Input: part model. Units: mm. Frame: model coordinates. A direction names the side the tool comes from. Coordinates: 2 decimals unless noted, no trailing zeros. Order: outer loops, then holes, each group sorted by start corner. A loop starts at its lowest first (then second) coordinate and runs counter-clockwise, first axis right, second up. Notation, with made-up numbers: (-24, 27) - (0, 27) arc R24 ccw to (0, 41) - close; hole circle Ø7 at (49.25, 66). An arc over 180 degrees is marked (long way). Use a Markdown table: item, result. Add a question column.
from build123d import *

# Parameters (mm, degrees)
F2_R     = 17.5
F3_DEPTH = 25
F5_SCALE = 0.5


with BuildPart() as f1:
    # F0 (on Front) → F1 (revolve)
    with BuildSketch(Plane.XZ):
        Polygon((0, 37.8452404466), (0, 0), (12.7, 0), (12.7, 52.3875), (4.4460149232, 52.3875), align=None)
        Polygon((0, 52.3875), (0, 37.8452404466), (4.4460149232, 52.3875), align=None)
        Polygon((9.20242, 67.945), (4.4460149232, 52.3875), (12.7, 52.3875), (12.7, 67.945), align=None)
    revolve(axis=Axis((21.4788783342, 0, 0), (1, 0, 0)))

    # F2 (on face) → F3 (cut)
    with BuildSketch(Plane(origin=(0, 0, 0), x_dir=(0, -1, 0), z_dir=(-1, 0, 0))):
        Circle(F2_R)
    extrude(amount=-F3_DEPTH, mode=Mode.SUBTRACT)

    # F4: F1 across plane


with BuildPart() as f1_1:
    add(f1.part)
    add(f1.part.mirror(Plane.YZ))


with BuildPart() as f1_2:
    # F5: moved
    add(f1_1.part.scale(F5_SCALE))


solid = f1_2.part
1) Pull-direction query (X, two-part tool) for faces 3 (the flat face through (-6.35, 7, -7)), 4 (the conical face through (-2.34, 25.94, -5.76)), 5 (the flat face through (6.35, 7, -7)); classes: pulls with the +X half, pulls with the -X half, needs draft (parallel to the pull), parting line crosses it, or undercut.
2) Cut plane D-D (x = -3). Return the cut outline in (y, z), and give its area (3 significant figures).
3) Cut plane A-A (z = 0). Return the cut outline in (x, y), and give its area (3 significant figures).
4) Reachability of faces 1 (the cylindrical face through (-5.463, -10.204, 32.404)), 2 (the conical face through (2.34, 25.94, -5.76)) from +Z, -Z, +X, -X, +Y, -Y: full face, straight path, thin tool, end or side. Return the list, or none.
5) Material intervals for L1, parallel to X at y = -23, z = 17.5; L2, parallel to X at y = -22.5, z = 24; L3, parallel to Z at x = 1.75, y = 3, sorted ascending.
6) Contact query for flat-ended pins moving along their axis: P1, Ø4, axis at x = -3, z = 0, coming from the -Y side; P2, Ø14, axis at y = 0, z = 0, coming from the +X side. Output: stop coordinate, or through.
Computed:
| question | item | result |
|---|---|---|
| 1 | face 3 | pulls with the -X half |
| 1 | face 4 | undercut |
| 1 | face 5 | pulls with the +X half |
| 2 | outline | circle Ø57.47 at (0, 0); hole circle Ø17.5 at (0, 0) |
| 2 | area | 2,350 mm2 |
| 3 | outline | (-6.35, -33.97) - (-4.6, -33.97) - (-2.22, -26.19) - (2.22, -26.19) - (4.6, -33.97) - (6.35, -33.97) - (6.35, -8.75) - (-6.35, -8.75) - close; (-6.35, 8.75) - (6.35, 8.75) - (6.35, 33.97) - (4.6, 33.97) - (2.22, 26.19) - (-2.22, 26.19) - (-4.6, 33.97) - (-6.35, 33.97) - close |
| 3 | area | 534 mm2 |
| 4 | face 1 | +X, -X |
| 4 | face 2 | none |
| 5 | L1 | x = -6.35 to -3.05, 3.05 to 6.35 |
| 5 | L2 | x = -6.35 to -4.27, 4.27 to 6.35 |
| 5 | L3 | z = -26.02 to -8.22, 8.22 to 26.02 |
| 6 | P1 | stops at y = -33.97 |
| 6 | P2 | passes through |
